```python
from build123d import *

# Parameters (mm, degrees)
SKETCH1_W          = 12.617819502
SKETCH1_H          = 2
SKETCH1_W_2        = 6.5532
SKETCH1_H_2        = 5.31
SKETCH2_R          = 1.0922
CUT_EXTRUDE1_DEPTH = 30.658943154
SKETCH3_W          = 45.123892984
SKETCH3_H          = 9
CUT_EXTRUDE2_DEPTH = 1


with BuildPart() as part:
    # Sketch1 → Revolve1 (revolve)
    with BuildSketch(Plane(origin=(0, 0, 0), x_dir=(1, 0, 0), z_dir=(0, 1, 0))):
        with Locations((-13.308909751, 3.700473465)):
            Rectangle(SKETCH1_W, SKETCH1_H)
        Polygon((-11.938, 2.700473465), (-19.617819502, 2.700473465), (-19.617819502, -0.474526535), (-13.064619502, -0.474526535), (-11.938, -0.474526535), align=None)
        with Locations((-16.341219502, -3.129526535)):
            Rectangle(SKETCH1_W_2, SKETCH1_H_2)
    revolve(axis=Axis((0, 0, -25.411285606), (0, 0, 1)))

    # Sketch2 → Cut-Extrude1 (cut, through all)
    with BuildSketch(Plane(origin=(0, 0, -4.700473465), x_dir=(-1, 0, 0), z_dir=(0, 0, -1))):
        with Locations((16.57, 0)):
            Circle(SKETCH2_R)
        with Locations(Location((-16.57, 0, 0), (0, 0, 180))):
            Circle(SKETCH2_R)
    extrude(amount=-CUT_EXTRUDE1_DEPTH, mode=Mode.SUBTRACT)

    # Sketch3 → Cut-Extrude2 (cut)
    with BuildSketch(Plane(origin=(0, 0, -4.700473465), x_dir=(-1, 0, 0), z_dir=(0, 0, -1))):
        Rectangle(SKETCH3_W, SKETCH3_H)
    extrude(amount=-CUT_EXTRUDE2_DEPTH, mode=Mode.SUBTRACT)


solid = part.part
```
Geometry check sheet. Reference: the model listing, model coordinates, mm. A direction names the side the tool comes from. Round coordinates to 2 decimals unless told otherwise and drop trailing zeros. Order: outer loops, then holes, each group sorted by start corner. A loop starts at its lowest first (then second) coordinate and runs counter-clockwise, first axis right, second up. Notation, with made-up numbers: (62, -7.75) - (94, -7.75) arc R35 cw to (94, 31.25) - close; hole circle Ø9 at (-24.75, 9). An arc over 180 degrees is marked (long way). Use a Markdown table: item, result. Add a question column.
1) Gauge pin test, flat ends, axial feed: P1, Ø8, axis at x = -2.5, y = -5, coming from the +Z side; P2, Ø4.5, axis at x = -10, y = -2, coming from the -Z side; P3, Ø3, axis at y = -12.5, z = 2.5, coming from the +X side. Record the tip position at first contact, or that the pin passes through.
2) Thickness scan on line 1 along Y through (x, z) = (0, -3.7); line 2 along Y through (x, z) = (-7.5, 1); line 3 along Z through (x, y) = (-9, -7.5). Record the ranges inside material, lowest first.
3) Mould release check, pull along X, two halves, no side actions. Record for faces 1 (the flat face through (12, -4.5, -4)), 2 (the cylindrical face through (-12.461, -3.924, 3.092)), 3 (the cylindrical face through (-18.712, -5.893, 0.615)): released by +X, released by -X, zero draft, split by the parting line, or undercut.
4) Section check D-D (y = 5.5). Record the cut outline in (x, z).
5) Section check C-C (z = -1.75). Record the cut outline in (x, y).
6) Section check A-A (x = 0). Record the cut outline in (y, z), then the cut area to 3 significant figures.
7) Set-up check for faces 4 (the flat face through (-6, 11, 0.475)), 5 (the flat face through (-4, 13, 5.785)), 6 (the flat face through (-12, -4.5, -4)): record each of +Z, -Z, +X, -X, +Y, -Y from which the full face is reachable in a straight line by a thin tool's end or side.
8) Section check B-B (y = 0). Record the cut outline in (x, z).
Established:
| question | item | result |
|---|---|---|
| 1 | P1 | z = -2.7 |
| 1 | P2 | z = -3.7 |
| 1 | P3 | x = 16.24 |
| 2 | line 1 | -19.62 to -7, 7 to 19.62 |
| 2 | line 2 | -18.13 to -10.7, 10.7 to 18.13 |
| 2 | line 3 | -4.7 to -2.7 |
| 3 | face 1 | zero draft |
| 3 | face 2 | undercut |
| 3 | face 3 | split by the parting line |
| 4 | outline | (-18.83, -4.7) - (-4.33, -4.7) - (-4.33, -2.7) - (-10.6, -2.7) - (-10.6, 0.47) - (-11.85, 0.47) - (-11.85, 5.78) - (-18.83, 5.78) - close; (4.33, -4.7) - (18.83, -4.7) - (18.83, 5.78) - (11.85, 5.78) - (11.85, 0.47) - (10.6, 0.47) - (10.6, -2.7) - (4.33, -2.7) - close |
| 5 | outline | circle Ø39.24 at (0, 0); hole circle Ø2.18 at (-16.57, 0); hole circle Ø23.88 at (0, 0); hole circle Ø2.18 at (16.57, 0) |
| 6 | outline | (-19.62, -4.7) - (-7, -4.7) - (-7, -2.7) - (-11.94, -2.7) - (-11.94, 0.47) - (-13.06, 0.47) - (-13.06, 5.78) - (-19.62, 5.78) - close; (7, -4.7) - (19.62, -4.7) - (19.62, 5.78) - (13.06, 5.78) - (13.06, 0.47) - (11.94, 0.47) - (11.94, -2.7) - (7, -2.7) - close |
| 6 | area | 169 mm2 |
| 7 | face 4 | +Z |
| 7 | face 5 | +Z, +X, -X, +Y, -Y |
| 7 | face 6 | -Z, +X, -X |
| 8 | outline | (-19.62, -3.7) - (-17.66, -3.7) - (-17.66, 5.78) - (-19.62, 5.78) - close; (-15.48, -3.7) - (-7, -3.7) - (-7, -2.7) - (-11.94, -2.7) - (-11.94, 0.47) - (-13.06, 0.47) - (-13.06, 5.78) - (-15.48, 5.78) - close; (7, -3.7) - (15.48, -3.7) - (15.48, 5.78) - (13.06, 5.78) - (13.06, 0.47) - (11.94, 0.47) - (11.94, -2.7) - (7, -2.7) - close; (17.66, -3.7) - (19.62, -3.7) - (19.62, 5.78) - (17.66, 5.78) - close |
